Model file for the job. Use its own axes, mm. A direction names the side the tool comes from. Give positions to 0.01 mm unless a question says otherwise; leave off trailing zeros. Loops run counter-clockwise (first coordinate to the right, second up) from the corner with the lowest first, then second, coordinate; pieces in that order, holes last. Notation, with made-up numbers: (-36.5, 70.5) - (-12.5, 70.5) arc R28 ccw to (-12.5, 89.5) - close; hole circle Ø11 at (-18.75, 50.5). An arc over 180 degrees is marked (long way). Use a Markdown table: item, result.
Autodesk Inventor part; units mm, degrees
ref_plane "Work Plane1" through (12.5, 0, 0) normal (1, 0, 0) x (0, 1, 0)
ref_plane "XZ Plane" through (0, 0, 0) normal (0, 1, 0) x (-1, 0, 0)
ref_plane "XY Plane" through (0, 0, 0) normal (0, 0, 1) x (1, 0, 0)
sketch "Sketch1" plane through (0, 0, 0) normal (0, 1, 0) x (-1, 0, 0)
  circle A0 centre (0, 0) radius 7.5
  circle A1 centre (0, 0) radius 3
  dimension "d0" = 15
  dimension "d1" = 6
extrude "Extrusion1" add sketch "Sketch1" along normal blind 17
sketch "Sketch2" plane through (0, 17, 0) normal (0, 1, 0) x (1, 0, 0)
  circle A0 centre (0, 0) radius 3
  circle A1 centre (0, 0) radius 2.75
  circle A2 centre (0, 0) radius 4
  dimension "d4" = 5.5
  dimension "d5" = 8
extrude "Extrusion2" add sketch "Sketch2" along normal blind 7 contours A2
fillet "Fillet1" radius 6 1 edges at (-4, 17, 0)
fillet "Fillet2" radius 6 2 edges at (0, 17, -7.5) (0, 17, 7.5)
ref_plane "Work Plane1" through (12.5, 0, 0) normal (1, 0, 0) x (0, 1, 0)
mirror "Mirror1" about plane through (12.5, 0, 0) normal (1, 0, 0) of "Extrusion1", "Extrusion2", "Fillet1", "Fillet2"
sketch "Sketch3" plane through (0, 0, 0) normal (0, 1, 0) x (-1, 0, 0)
  circle A0 centre (-25, 0) radius 3
  line L0 (-25, 0) -> (-25, 3)
  line L1 (-25, 0) -> (-25, -3)
  line L2 (0, 0) -> (0, -3)
  circle A1 centre (0, 0) radius 3
  line L3 (0, 0) -> (0, 3)
  line L4 (-25, 3) -> (0, 3)
  line L5 (0, 3) -> (0, 7.5)
  line L6 (0, 7.5) -> (-25, 7.5)
  line L7 (-25, 7.5) -> (-25, 3)
  line L8 (-25, -3) -> (0, -3)
  line L9 (0, -3) -> (0, -7.5)
  line L10 (0, -7.5) -> (-25, -7.5)
  line L11 (-25, -7.5) -> (-25, -3)
  point P0 (0, -3)
  point P1 (0, 3)
  dimension "d11" = 25
  dimension "d12" = 4.5
  dimension "d13" = 25
  dimension "d14" = 4.5
extrude "Extrusion3" add sketch "Sketch3" along normal blind 11 contours A0 L4 A1 L8 | L7 L6 L5 L4 | L8 L9 L10 L11
sketch "Sketch4" plane through (0, 0, 7.5) normal (0, 0, 1) x (1, 0, 0)
  line L0 (25, 11) -> (0, 11)
  line L1 (12.5, 11) -> (12.5, 6)
  circle A0 centre (12.5, 6) radius 3
  point P0 (0, 0)
  dimension "d17" = 5
  dimension "d18" = 6
extrude "Extrusion4" cut sketch "Sketch4" against normal through all
properties part number "4mm_Roller_Spacer_simple"
(1) Pin check, flat tips, straight feed: P1, Ø8, axis at x = 18, y = 13, coming from the +Z side; P2, Ø5, axis at x = 12.5, y = 6, coming from the -Z side; P3, Ø3, axis at y = 20, z = 0, coming from the -X side; P4, Ø1, axis at y = 11.5, z = 5, coming from the -X side. Stop position of each tip, or through.
Computed:
| item | result |
|---|---|
| P1 | z = 7.5 |
| P2 | through |
| P3 | x = -5.49 |
| P4 | x = -6 |
(2) Drill centre lines: probe 1 along X at (y, z) = (9.25, 0); probe 2 along X at (y, z) = (14, 0); probe 3 along Y at (x, z) = (12.5, 3.75). Where is each one in solid material? Low to high. Write a range as [from, to].
Computed:
| item | result |
|---|---|
| probe 1 | [-7.5, -3], [3, 22], [28, 32.5] |
| probe 2 | [-7.5, -3], [3, 7.5], [17.5, 22], [28, 32.5] |
| probe 3 | [0, 3], [9, 11] |
(3) Slice it at B-B, the plane x = 12.5. Write the cut outline in (y, z), plus the area to 3 significant figures.
Computed:
| item | result |
|---|---|
| outline | (0, -7.5) - (3, -7.5) - (3, 7.5) - (0, 7.5) - close; (9, -7.5) - (11, -7.5) - (11, 7.5) - (9, 7.5) - close |
| area | 75.0 mm² |
(4) 3-axis set-ups, long thin cutter, end or side, ignore diameter. For faces 4 (the cylindrical face through (-7.154, 8.448, -2.253)), 5 (the flat face through (26, 24, -3)): which of +Z, -Z, +X, -X, +Y, -Y reach the whole face in a straight line?
Computed:
| item | result |
|---|---|
| face 4 | +Y |
| face 5 | +Z, -Z, +X, -X, +Y |
(5) Mould opens along X. For faces 1 (the cylindrical face through (28.2, 23.2, 2.4)), 2 (the flat face through (13, 0, 0)), 3 (the flat face through (13, 11, 0)) say: pulls with the +X half, pulls with the -X half, needs draft (parallel to the pull), parting line crosses it, or undercut.
Computed:
| item | result |
|---|---|
| face 1 | undercut |
| face 2 | needs draft |
| face 3 | undercut |
(6) Slice it at C-C, the plane y = 9.75. Write the cut outline in (x, z), plus the area to 3 significant figures.
Computed:
| item | result |
|---|---|
| outline | (0, -7.5) - (25, -7.5) arc R7.5 ccw to (25, 7.5) - (0, 7.5) arc R7.5 ccw to start; hole circle Ø6 at (0, 0); hole circle Ø6 at (25, 0) |
| area | 495 mm² |
(7) Slice it at A-A, the plane y = 6. Write the cut outline in (x, z), plus the area to 3 significant figures.
Computed:
| item | result |
|---|---|
| outline | (0, -7.5) - (9.5, -7.5) - (9.5, 7.5) - (0, 7.5) arc R7.5 ccw to start; (15.5, -7.5) - (25, -7.5) arc R7.5 ccw to (25, 7.5) - (15.5, 7.5) - close; hole circle Ø6 at (0, 0); hole circle Ø6 at (25, 0) |
| area | 405 mm² |
(8) Slice it at D-D, the plane z = -2.25. Count the separate pieces of the cut face and the enclosed holes in it, plus the area to 3 significant figures.
Computed:
| item | result |
|---|---|
| separate pieces | 3 |
| enclosed holes | 1 |
| area | 498 mm² |
